CAD build for the part. Positions are in the model's coordinates, mm. A direction names the side the tool comes from. Give positions to 0.01 mm unless a question says otherwise; leave off trailing zeros. Order: outer loops, then holes, each group sorted by start corner. A loop starts at its lowest first (then second) coordinate and runs counter-clockwise, first axis right, second up. Notation, with made-up numbers: M 9,39.25 L 57,39.25 A15 ccw 57,60.25 Z; hole C -21,77.5 d7. An arc over 180 degrees is marked long. Put each result on its own line as item: value. Start each with the question number.
1) Drill centre lines: line 1 (X direction, y = 3, z = -19); line 2 (X direction, y = 39, z = 25); line 3 (Z direction, x = -1, y = 8.5). Where is each one in solid material? Low to high. Write a range as [from, to].
2) Tool access for faces 4 (the face through (-4.43, 35.49, 29.4)), 5 (the face through (5, 35, 2)), 6 (the face through (-0.07, 30.42, 26.5)): list every direction of +Z, -Z, +X, -X, +Y, -Y with a clear straight run to the whole face (end or side of a thin tool).
3) Two-plate mould, pull along Z, no slides. Class faces 1 (the face through (44.68, 30.42, -54.6)), 2 (the face through (-5, 35, -1)), 3 (the face through (46.768, 35.49, -59.194)): released by +Z, released by -Z, zero draft, split by the parting line, or undercut.
4) Cut at A-A (y = 26.5). Write the cut outline in (x, z), and give its area (3 significant figures).
5) Cut at B-B (z = 3). Write the cut outline in (x, y).
6) Cut at C-C (x = 27). Write the cut outline in (y, z), and give its area (3 significant figures).
7) Pin check, flat tips, straight feed: pin 1 (5 mm diameter, centred on x = 36, y = 18.5, fed in from -Z); pin 2 (1 mm diameter, centred on x = 43, y = 58, fed in from +Z); pin 3 (2.5 mm diameter, centred on x = 0, z = 25, fed in from -Y). Stop position of each tip, or through.
Autodesk Inventor part; units mm, degrees
ref_plane "YZ Plane" through (0, 0, 0) normal (1, 0, 0) x (0, 1, 0)
ref_plane "XZ Plane" through (0, 0, 0) normal (0, 1, 0) x (-1, 0, 0)
ref_plane "XY Plane" through (0, 0, 0) normal (0, 0, 1) x (1, 0, 0)
sketch "Эскиз1" plane through (0, 0, 0) normal (0, 1, 0) x (-1, 0, 0)
  line L0 (16.3923, 0) -> (-63.3538, 0) construction
  line L1 (5, 30) -> (-5, 30)
  line L2 (5, -30) -> (5, 30)
  line L3 (5, -30) -> (-46.9615, -60)
  line L4 (-46.9615, -60) -> (-51.9615, -51.3397)
  line L5 (-51.9615, -51.3397) -> (-5, -24.2265)
  line L6 (-5, -24.2265) -> (-5, 30)
  line L7 (0, -78) -> (0, 48) construction
  point P0 (0, 0)
  dimension "d13" = 60
  dimension "d16" = 10
  dimension "d17" = 10
  dimension "d18" = 60
  dimension "d19" = 120
extrude "Выдавливание1" add sketch "Эскиз1" along normal blind 70
fillet "Сопряжение1" radius 2 6 edges at (-5, 35, 30) (5, 35, 30) (-5, 35, -30) (51.9615, 35, -51.3397) (46.9615, 35, -60) (5, 35, -24.2265)
sketch "Эскиз7" plane through (0, 0, 0) normal (0, -1, 0) x (1, 0, 0)
  line L0 (-3, 30) -> (3, 30)
  line L1 (5, 28) -> (5, -23.0718)
  line L2 (6, -24.8038) -> (50.2295, -50.3397)
  line L3 (50.9615, -53.0718) -> (47.9615, -58.2679)
  point P0 (0, 0)
  point P1 (0, 25)
  point P2 (45.1314, -53.1699)
  dimension "d21" = 5
  dimension "d22" = 5
  dimension "d23" = 5
  dimension "d24" = 5
hole "Отверстие1" at (0, 0, 25) at (45.1314, 0, -53.1699) direction (0, 1, 0) diameter 3 depth 60 tip angle 118
properties part number "Лепесток БСП"
Solution:
1. line 1: [-5, 5]
1. line 2: [-5, -1.5], [1.5, 5]
1. line 3: [-32.31, 23.88], [26.12, 30]
2. face 4: +Z, -X, +Y, -Y
2. face 5: +Z, +X, +Y, -Y
2. face 6: -Y
3. face 1: undercut
3. face 2: zero draft
3. face 3: released by -Z
4. outline: M -5,-28.85 A2 ccw -4,-30.58 L 45.23,-59 A2 ccw 47.96,-58.27 L 50.96,-53.07 A2 ccw 50.23,-50.34 L 6,-24.8 A2 cw 5,-23.07 L 5,28 A2 ccw 3,30 L -3,30 A2 ccw -5,28 Z; hole C 0,25 d3; hole C 45.13,-53.17 d3
4. area: 1,120 mm²
5. outline: M -5,0 L 5,0 L 5,70 L -5,70 Z
6. outline: M 0,-48.48 L 70,-48.48 L 70,-36.93 L 0,-36.93 Z
6. area: 808 mm²
7. pin 1: z = -55.11
7. pin 2: z = -45.88
7. pin 3: y = 60.15
